Geometry check sheet. Reference: the model listing, model coordinates, mm. A direction names the side the tool comes from. Round coordinates to 2 decimals unless told otherwise and drop trailing zeros. Loops run counter-clockwise (first coordinate to the right, second up) from the corner with the lowest first, then second, coordinate; pieces in that order, holes last. Notation, with made-up numbers: M 25.25,2 L 43.25,2 A18 ccw 43.25,30 Z; hole C 2.5,39.25 d3. An arc over 180 degrees is marked long. Write item = value, one per line.
from build123d import *

# Parameters (mm, degrees)
SKETCH_2_R          = 1.5
EXTRUDE_1_DEPTH     = 10
SKETCH_2_3_R        = 1.5
CUT_EXTRUDE_1_DEPTH = 4.5
SKETCH_3_R          = 5.5
EXTRUDE_2_DEPTH     = 11.5
SKETCH_4_R          = 3
CUT_EXTRUDE_2_DEPTH = 9.5


with BuildPart() as part:
    # Sketch 2 → Extrude 1 (new body)
    # profile 1 of 2: a face of its own
    with BuildSketch(Plane(origin=(0, 0, 0), x_dir=(0, 0, -1), z_dir=(1, 0, 0))):
        Polygon((0.986233019, -3.680671736), (3.680671736, -0.986233019), (2.694438717, 2.694438717), (-0.986233019, 3.680671736), (-3.680671736, 0.986233019), (-2.694438717, -2.694438717), align=None)
        Circle(SKETCH_2_R, mode=Mode.SUBTRACT)
    # profile 2 of 2: a face of its own
    with BuildSketch(Plane(origin=(0, 0, 0), x_dir=(0, 0, -1), z_dir=(1, 0, 0))):
        Circle(SKETCH_2_R)
    extrude(amount=EXTRUDE_1_DEPTH)

    # Sketch 2_3 → Cut-Extrude 1 (cut)
    with BuildSketch(Plane(origin=(0, 0, 0), x_dir=(0, 0, -1), z_dir=(1, 0, 0))):
        Circle(SKETCH_2_3_R)
    extrude(amount=CUT_EXTRUDE_1_DEPTH, mode=Mode.SUBTRACT)

    # Sketch 3 → Extrude 2 (add)
    with BuildSketch(Plane(origin=(10, 0, 0), x_dir=(0, 0, -1), z_dir=(1, 0, 0))):
        Circle(SKETCH_3_R)
    extrude(amount=EXTRUDE_2_DEPTH)

    # Sketch 4 → Cut-Extrude 2 (cut)
    with BuildSketch(Plane(origin=(21.5, 0, 0), x_dir=(0, 0, -1), z_dir=(1, 0, 0))):
        Circle(SKETCH_4_R)
    extrude(amount=-CUT_EXTRUDE_2_DEPTH, mode=Mode.SUBTRACT)


solid = part.part
(1) Sectioned sample at D-D on x = 15.75. Record the cut outline in (y, z).
Result set:
outline = C 0,0 d11; hole C 0,0 d6
(2) Material ranges on line 1 along Y through (x, z) = (19, 0); line 2 along X through (y, z) = (-3.75, 2.75); line 3 along Y through (x, z) = (14, 0.75), recorded low to high. Write a range as from..to.
Result set:
line_1 = -5.5..-3, 3..5.5
line_2 = 10..21.5
line_3 = -5.45..-2.9, 2.9..5.45
(3) Sectioned sample at A-A on x = 5.75. Record the cut outline in (y, z), then the cut area to 3 significant figures.
Result set:
outline = M -3.68,-0.99 L -0.99,-3.68 L 2.69,-2.69 L 3.68,0.99 L 0.99,3.68 L -2.69,2.69 Z
area = 37.7 mm2
(4) Release check for a two-part mould opening along Y. For faces 6 (the cylindrical face through (17, 0, 3)), 7 (the flat face through (0, 0, -2)), 8 (the flat face through (4.93, -2.352, -2.315)) record: released by +Y, released by -Y, zero draft, split by the parting line, or undercut.
Result set:
face_6 = undercut
face_7 = zero draft
face_8 = released by -Y
(5) Depth check by flat-ended pin: pin 1 Ø1.5 at (x, y) = (6.5, -2.5) entering from +Z; pin 2 Ø4 at (x, z) = (4.5, -3.5) entering from +Y; pin 3 Ø4 at (x, y) = (8.5, -4.5) entering from -Z. Enter the tip coordinate at first touch or a pass-through.
Result set:
pin_1 = 2.95
pin_2 = 3.01
pin_3 = -4.49
(6) Tool access check on faces 1 (the flat face through (12, 0, 0)), 2 (the flat face through (4.9, 0.8, -3.2)), 3 (the flat face through (4.5, 0, 0)), 4 (the flat face through (4.9, -0.8, 3.2)), 5 (the flat face through (4.93, 2.352, 2.315)). Record the directions out of +Z, -Z, +X, -X, +Y, -Y that give a thin tool (end or side, any length) a straight path to the whole face; none if there is none.
Result set:
face_1 = +X
face_2 = -Z, -X, +Y
face_3 = -X
face_4 = +Z, -X, -Y
face_5 = +Z, -X, +Y
(7) Sectioned sample at C-C on y = 3.25. Record the cut outline in (x, z), then the cut area to 3 significant figures.
Result set:
outline = M 0,-0.62 L 10,-0.62 L 10,-4.44 L 21.5,-4.44 L 21.5,4.44 L 10,4.44 L 10,1.42 L 0,1.42 Z
area = 122 mm2
(8) Sectioned sample at B-B on z = 0.75. Record the cut outline in (x, y).
Result set:
outline = M 0,-3.22 L 10,-3.22 L 10,-5.45 L 21.5,-5.45 L 21.5,-2.9 L 12,-2.9 L 12,2.9 L 21.5,2.9 L 21.5,5.45 L 10,5.45 L 10,3.62 L 0,3.62 L 0,1.3 L 4.5,1.3 L 4.5,-1.3 L 0,-1.3 Z
